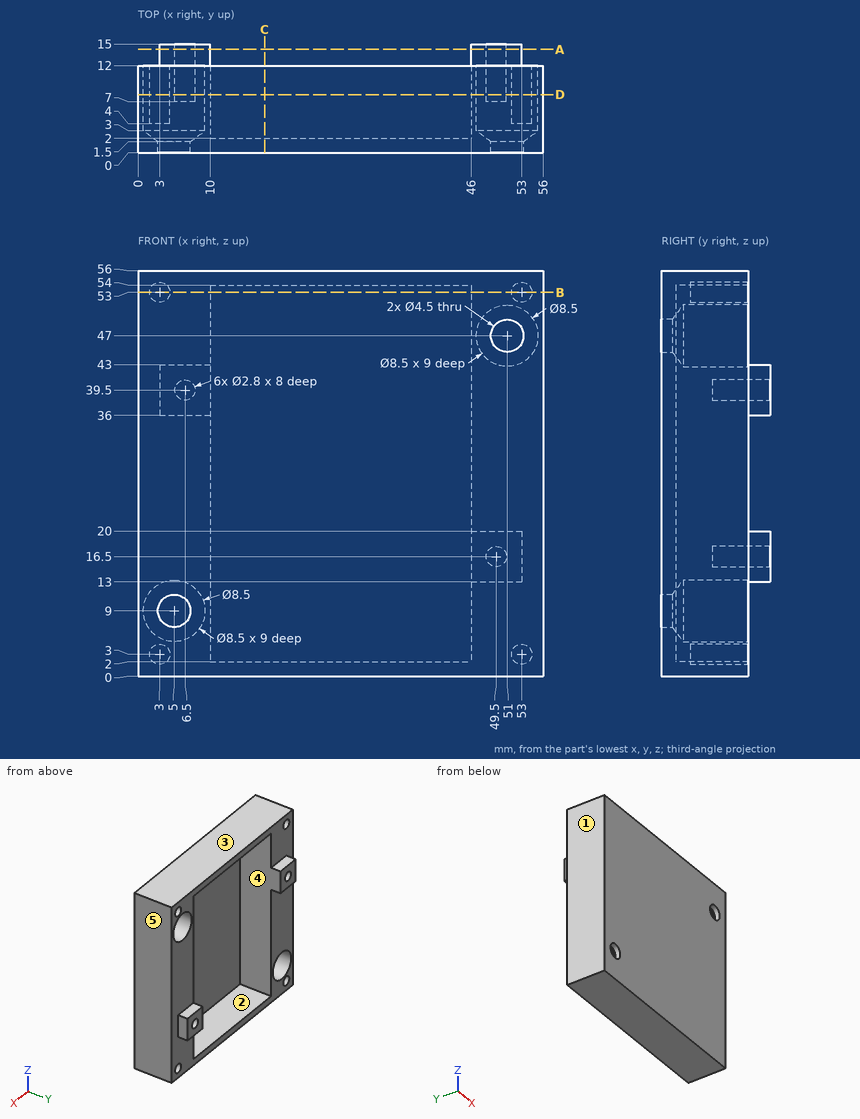
Print and shaded views of the part. All mm, measured from the part's lowest x, y and z. A direction names the side the tool comes from. Give positions to 0.01 mm unless a question says otherwise; leave off trailing zeros. Loops run counter-clockwise (first coordinate to the right, second up) from the corner with the lowest first, then second, coordinate; pieces in that order, holes last. Notation, with made-up numbers: (66, -22.75) - (121, -22.75) arc R23 cw to (121, 16.25) - close; hole circle Ø2 at (-32, -21.5). An arc over 180 degrees is marked (long way). Use a Markdown table: item, result.
(1) Band-saw the part on D-D (y = 8). Give the number of separate pieces and of enclosed holes in the cut face, and give its area (3 significant figures).
Taken from the geometry:
| item | result |
|---|---|
| separate pieces | 1 |
| enclosed holes | 9 |
| area | 1,110 mm2 |
(2) Pull direction X, two halves, no side cores. Call the marked faces 3, 4 and 5: +X half, -X half, draft (parallel to the pull), parting line (faces both ways), or undercut.
Taken from the geometry:
| item | result |
|---|---|
| face 3 | draft |
| face 4 | undercut |
| face 5 | +X half |
(3) Band-saw the part on C-C (x = 17.5). Give the cut face in (y, z).
Taken from the geometry:
| item | result |
|---|---|
| outline | (0, 0) - (12, 0) - (12, 2) - (2, 2) - (2, 54) - (12, 54) - (12, 56) - (0, 56) - close |
(4) Band-saw the part on A-A (y = 14.25). Give the cut face in (x, z), and give its area (3 significant figures).
Taken from the geometry:
| item | result |
|---|---|
| outline | (3, 36) - (10, 36) - (10, 43) - (3, 43) - close; (46, 13) - (53, 13) - (53, 20) - (46, 20) - close; hole circle Ø2.8 at (6.5, 39.5); hole circle Ø2.8 at (49.5, 16.5) |
| area | 85.7 mm2 |
(5) Which spindle directions (+Z, -Z, +X, -X, +Y, -Y) get a long thin tool onto all of the face, cutting with end or side? Do the marked faces 1 and 2. Say none if no direction does.
Taken from the geometry:
| item | result |
|---|---|
| face 1 | +Z, -Z, -X, +Y, -Y |
| face 2 | +Y |
(6) Drop flat-ended pins along their axis: pin 1 Ø1.4 at (x, z) = (3, 3.5) entering from +Y; pin 2 Ø3 at (x, z) = (53, 52.5) entering from +Y; pin 3 Ø1.5 at (x, y) = (49, 13.5) entering from +Z. Give the stop position or say it passes through.
Taken from the geometry:
| item | result |
|---|---|
| pin 1 | y = 4 |
| pin 2 | y = 12 |
| pin 3 | z = 20 |
(7) Band-saw the part on B-B (z = 53). Give the cut face in (x, y).
Taken from the geometry:
| item | result |
|---|---|
| outline | (0, 0) - (56, 0) - (56, 12) - (54.4, 12) - (54.4, 4) - (51.6, 4) - (51.6, 12) - (46, 12) - (46, 2) - (10, 2) - (10, 12) - (4.4, 12) - (4.4, 4) - (1.6, 4) - (1.6, 12) - (0, 12) - close |
(8) Wall check: line 1 along X through (y, z) = (11.5, 15); line 2 along Z through (x, y) = (26, 11.5); line 3 along X through (y, z) = (5.5, 52). Give the ranges that are in metal, low to high.
Taken from the geometry:
| item | result |
|---|---|
| line 1 | 0 to 10, 46 to 56 |
| line 2 | 0 to 2, 54 to 56 |
| line 3 | 0 to 2.02, 3.98 to 10, 46 to 52.02, 53.98 to 56 |
